```python
from build123d import *

# Parameters (mm, degrees)
F0_W     = 50
F0_H     = 50
F1_DEPTH = 5
F2_W     = 15
F2_H     = 25
F3_DEPTH = 169
F4_DEPTH = 17
F5_DEPTH = 41
F6_W     = 15
F6_H     = 25
F7_DEPTH = 141


with BuildPart() as f1:
    # F0 (on Top) → F1 (new body)
    with BuildSketch(Plane.XY):
        Rectangle(F0_W, F0_H)
    extrude(amount=F1_DEPTH)

    # F2 (on face) → F3 (cut)
    with BuildSketch(Plane.XY.offset(5)):
        Rectangle(F2_W, F2_H)
    extrude(amount=-F3_DEPTH, mode=Mode.SUBTRACT)

    # F4 (add): a face of the model
    f4_faces = [f1.faces().sort_by_distance(p)[0] for p in [
        (0, -24.2928932188, 5),
    ]]
    extrude(f4_faces, amount=F4_DEPTH)

    # F5 (add): a face of the model
    f5_faces = [f1.faces().sort_by_distance(p)[0] for p in [
        (0, -25, 11),
    ]]
    extrude(f5_faces, amount=F5_DEPTH)

    # F6 (on face) → F7 (cut)
    with BuildSketch(Plane.XY.offset(22)):
        with Locations((0, -40.7508090138)):
            Rectangle(F6_W, F6_H)
    extrude(amount=-F7_DEPTH, mode=Mode.SUBTRACT)


solid = f1.part
```
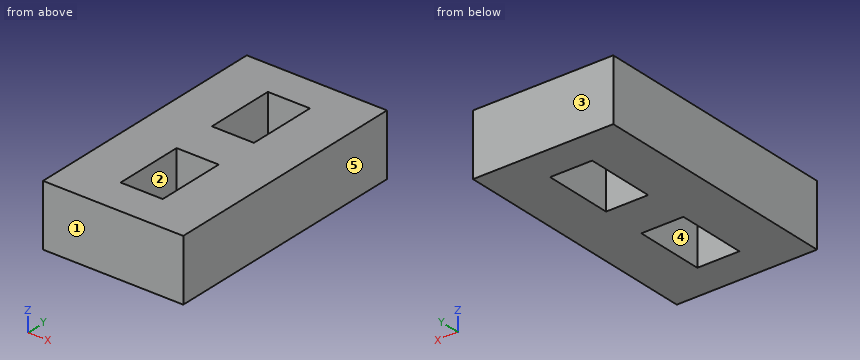
The model under review builds one solid part; all positions refer to its coordinate system, in mm. Face numbers are marked on the shaded views. A direction names the side the tool comes from. Give positions to 0.01 mm unless a question says otherwise; leave off trailing zeros. Order: outer loops, then holes, each group sorted by start corner. A loop starts at its lowest first (then second) coordinate and runs counter-clockwise, first axis right, second up. Notation, with made-up numbers: (24.25, 29) - (46.25, 29) arc R20 cw to (46.25, 41) - close; hole circle Ø11 at (61.5, -38). An arc over 180 degrees is marked (long way). Use CSV: the item, a comma, the result in double quotes. Start each with the question number.
Q1. We need section A-A, the plane x = -1.5. Write out the cut boundary in (y, z).
Q2. To check wall thickness, follow line 1 along Y through (x, z) = (0.5, 11.5); line 2 along X through (y, z) = (1.5, 4.75). State the ranges of each line that lie inside material, in increasing order. Write a range as [from, to].
Q3. Tool access review of the marked faces 1 and 2: name each direction out of +Z, -Z, +X, -X, +Y, -Y from which nothing blocks a thin tool from reaching the whole face with its end or side.
Q4. We need section C-C, the plane y = -4.5. Write out the cut boundary in (x, z), and give its area (3 significant figures).
Q5. The part is to be moulded in two halves that separate along Y. For the marked faces 3, 4 and 5, say which applies: +Y half, -Y half, draft (parallel to the pull), parting line (faces both ways), or undercut.
Q6. We need section B-B, the plane z = 9.5. Write out the cut boundary in (x, y), and give its area (3 significant figures).
Outcome:
1,outline,"(-66, 0) - (-53.25, 0) - (-53.25, 22) - (-66, 22) - close; (-28.25, 0) - (-12.5, 0) - (-12.5, 22) - (-28.25, 22) - close; (12.5, 0) - (25, 0) - (25, 22) - (12.5, 22) - close"
2,line 1,"y = [-66, -53.25], [-28.25, -12.5], [12.5, 25]"
2,line 2,"x = [-25, -7.5], [7.5, 25]"
3,face 1,"+Z, -Z, +X, -X, -Y"
3,face 2,"+Z, -Z"
4,outline,"(-25, 0) - (-7.5, 0) - (-7.5, 22) - (-25, 22) - close; (7.5, 0) - (25, 0) - (25, 22) - (7.5, 22) - close"
4,area,"770 mm^2"
5,face 3,"+Y half"
5,face 4,"undercut"
5,face 5,"draft"
6,outline,"(-25, -66) - (25, -66) - (25, 25) - (-25, 25) - close; hole (-7.5, -53.25) - (7.5, -53.25) - (7.5, -28.25) - (-7.5, -28.25) - close; hole (-7.5, -12.5) - (7.5, -12.5) - (7.5, 12.5) - (-7.5, 12.5) - close"
6,area,"3,800 mm^2"
